```python
from build123d import *

# Parameters (mm, degrees)
ESBO_O1_R                = 22.5
RESSALTO_EXTRUS_O1_DEPTH = 10
ESBO_O3_W                = 70
ESBO_O3_H                = 60
RESSALTO_EXTRUS_O2_DEPTH = 6.5
ESBO_O5_R                = 5
RESSALTO_EXTRUS_O3_DEPTH = 13
CHANFRO1_SIZE            = 0.5
FILETE1_R                = 5


# Read off the part's stored shape, not the designer's step: Varredura1
with BuildPart() as part:
    # Esboço1 → Ressalto-extrusão1 (new body)
    with BuildSketch(Plane(origin=(0, 0, 0), x_dir=(1, 0, 0), z_dir=(0, 1, 0))):
        with Locations(Location((0, 0, 0), (0, 0, 270))):
            Circle(ESBO_O1_R)
    extrude(amount=RESSALTO_EXTRUS_O1_DEPTH)

    # Esboço3 → Ressalto-extrusão2 (add)
    with BuildSketch(Plane(origin=(0, 10, 0), x_dir=(1, 0, 0), z_dir=(0, 1, 0))):
        Rectangle(ESBO_O3_W, ESBO_O3_H)
    extrude(amount=RESSALTO_EXTRUS_O2_DEPTH)

    # Varredura1 outline → Varredura1 (revolve)
    with BuildSketch(Plane.XY):
        with BuildLine():
            Line((22.5, 2.5), (22.5, 0))
            ThreePointArc((22.5, 0), (23.75, 1.25), (22.5, 2.5))
        make_face()
    revolve(axis=Axis((0, 0, 0), (0, 1, 0)))

    # Esboço5 → Ressalto-extrusão3 (add)
    with BuildSketch(Plane.XZ):
        with Locations(Location((0, 0, 0), (0, 0, 90))):
            Circle(ESBO_O5_R)
    extrude(amount=RESSALTO_EXTRUS_O3_DEPTH)

    # Chanfro1
    chanfro1_edges = [part.edges().sort_by_distance(p)[0] for p in [
        (0, -13, -5),
    ]]
    chamfer(chanfro1_edges, length=CHANFRO1_SIZE)

    # Filete1
    filete1_edges = [part.edges().sort_by_distance(p)[0] for p in [
        (35, 13.25, 30),
        (35, 13.25, -30),
        (-35, 13.25, -30),
        (-35, 13.25, 30),
    ]]
    fillet(filete1_edges, radius=FILETE1_R)


solid = part.part
```
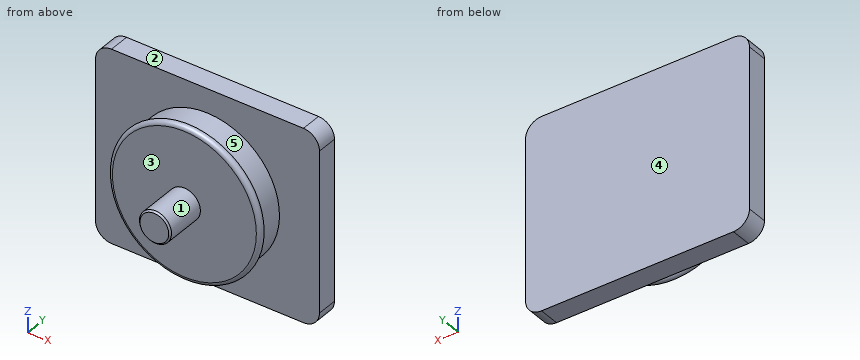
For this review, take the finished solid that the model builds, in its own axes (mm). Face numbers are marked on the shaded views. A direction names the side the tool comes from. Coordinates: 2 decimals unless noted, no trailing zeros. Order: outer loops, then holes, each group sorted by start corner. A loop starts at its lowest first (then second) coordinate and runs counter-clockwise, first axis right, second up. Notation, with made-up numbers: (87, -14.75) -> (99, -14.75) arc R18 cw to (99, -4.75) -> close; hole circle Ø7 at (33.5, 85.25). An arc over 180 degrees is marked (long way). Use CSV: the item, a comma, the result in double quotes. Start each with the question number.
Item 1: Wall thickness on probe 1 along Y at (x, z) = (-29, 20.5); probe 2 along Y at (x, z) = (-12, -4.5); probe 3 along Z at (x, y) = (-3.5, 4.75): over which ranges is each line inside the solid? List them lowest first.
Item 2: For the marked faces 1 and 2, list the 3-axis set-ups (+Z, -Z, +X, -X, +Y, -Y) from which the entire face can be reached by the end or side of a thin tool; tool diameter is ignored.
Item 3: We need section D-D, the plane z = -26. Give the boundary of the cut face in (x, y).
Item 4: We need section C-C, the plane y = -5.5. Give the boundary of the cut face in (x, z), then the cut area to 3 significant figures.
Item 5: We need section B-B, the plane x = 0. Give the boundary of the cut face in (y, z).
Item 6: Insertion check: pin 1 (22.5 mm diameter, centred on x = -10.5, z = 0.5, fed in from -Y); pin 2 (2 mm diameter, centred on x = 11, z = 12.5, fed in from -Y); pin 3 (1 mm diameter, centred on y = 6.5, z = -16.5, fed in from -X); pin 4 (8 mm diameter, centred on y = -3, z = -5.5, fed in from -X). Each pin has a flat end and moves straight along its axis. Give the tip position at first contact, or say it passes through.
Item 7: We need section A-A, the plane z = 0. Give the boundary of the cut face in (x, y), then the cut area to 3 significant figures.
Item 8: Draft analysis for pull direction Y (two halves, no side actions). For the marked faces 3, 4 and 5, state which applies: pulls with the +Y half, pulls with the -Y half, needs draft (parallel to the pull), parting line crosses it, or undercut.
Derived:
1,probe 1,"y = 10 to 16.5"
1,probe 2,"y = 0 to 16.5"
1,probe 3,"z = -22.23 to 22.23"
2,face 1,"-Y"
2,face 2,"+Z, +X, -X, +Y, -Y"
3,outline,"(-34.9, 10) -> (34.9, 10) -> (34.9, 16.5) -> (-34.9, 16.5) -> close"
4,outline,"circle Ø10 at (0, 0)"
4,area,"78.5 mm^2"
5,outline,"(-13, -4.5) -> (-12.5, -5) -> (0, -5) -> (0, -22.5) arc R1.25 ccw to (2.5, -22.5) -> (10, -22.5) -> (10, -30) -> (16.5, -30) -> (16.5, 30) -> (10, 30) -> (10, 22.5) -> (2.5, 22.5) arc R1.25 ccw to (0, 22.5) -> (0, 5) -> (-12.5, 5) -> (-13, 4.5) -> close"
6,pin 1,"stops at y = -13"
6,pin 2,"stops at y = 0"
6,pin 3,"stops at x = -15.82"
6,pin 4,"stops at x = -23.29"
7,outline,"(-35, 10) -> (-22.5, 10) -> (-22.5, 2.5) arc R1.25 ccw to (-22.5, 0) -> (-5, 0) -> (-5, -12.5) -> (-4.5, -13) -> (4.5, -13) -> (5, -12.5) -> (5, 0) -> (22.5, 0) arc R1.25 ccw to (22.5, 2.5) -> (22.5, 10) -> (35, 10) -> (35, 16.5) -> (-35, 16.5) -> close"
7,area,"1,040 mm^2"
8,face 3,"pulls with the -Y half"
8,face 4,"pulls with the +Y half"
8,face 5,"undercut"
